Source: three-view drawing plus pictorial views. Frame: mm from the lowest corner of the part. Coordinates: 2 decimals unless noted, no trailing zeros. Loops run counter-clockwise (first coordinate to the right, second up) from the corner with the lowest first, then second, coordinate; pieces in that order, holes last. Notation, with made-up numbers: M 43,-1.75 L 100,-1.75 A13 cw 100,16.25 Z; hole C -19,75.5 d8. An arc over 180 degrees is marked long. Write each question's results on one line, items separated by ' | '. Start each with the question number.
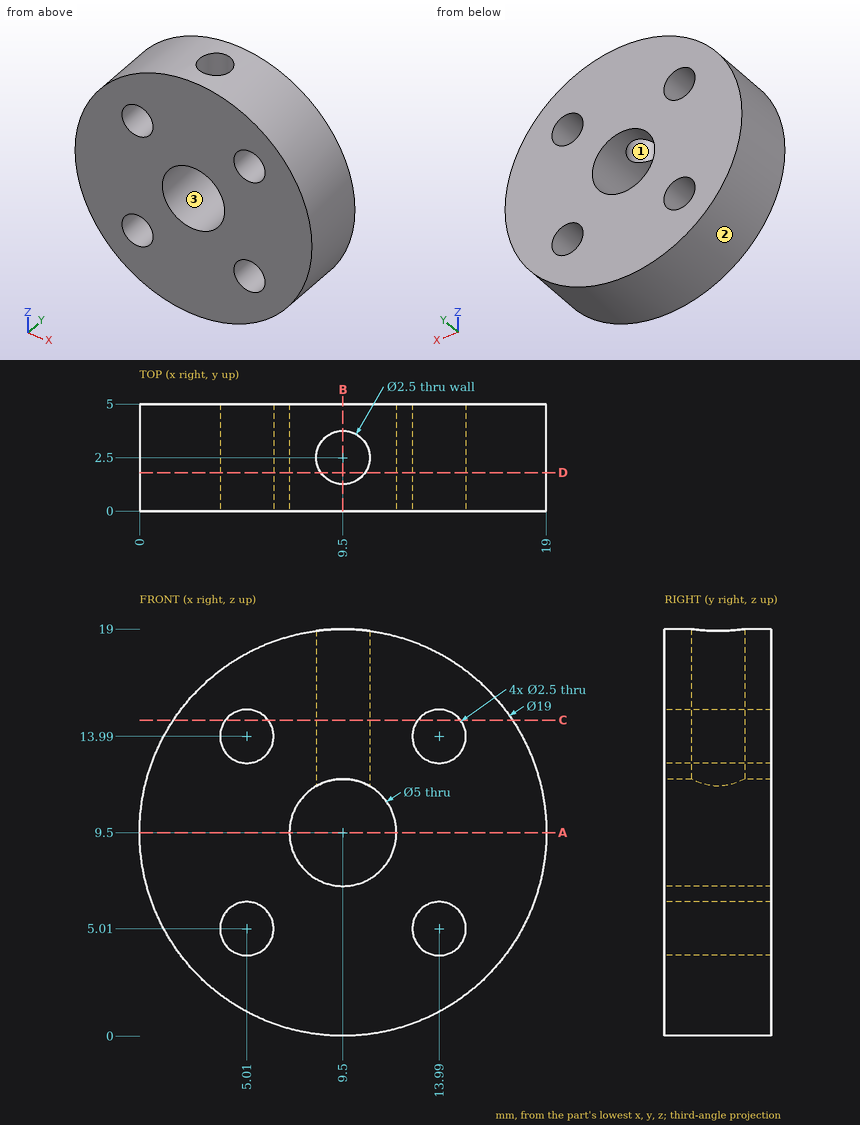
Item 1: Ray query, L1, parallel to Y at x = 9.5, z = 16.75; L2, parallel to X at y = 2.75, z = 5.75. Return the intervals inside material, ascending. Write a range as [from, to].
Item 2: Section D-D, the plane y = 1.8. Return loops of the section in (x, z), plus the area to 3 significant figures.
Item 3: Section B-B, the plane x = 9.5. Return loops of the section in (y, z), plus the area to 3 significant figures.
Item 4: Contact query for flat-ended pins moving along their axis: P1, Ø2, axis at x = 14.5, y = 4, coming from the +Z side; P2, Ø2, axis at x = 15.5, y = 1, coming from the +Z side. Output: stop coordinate, or through.
Item 5: Pull-direction query (Z, two-part tool) for the marked faces 1, 2 and 3; classes: released by +Z, released by -Z, zero draft, split by the parting line, or undercut.
Item 6: Section C-C, the plane z = 14.75. Return loops of the section in (x, y), plus the area to 3 significant figures.
Item 7: Section A-A, the plane z = 9.5. Return loops of the section in (x, y).
Solutions:
1) L1: y = [0, 1.25], [3.75, 5] | L2: x = [0.77, 4], [6.02, 12.98], [15, 18.23]
2) outline: M 8.46,11.78 L 8.46,18.94 A9.5 ccw long 10.54,18.94 L 10.54,11.78 A2.5 cw long Z; hole C 5.01,5.01 d2.5; hole C 5.01,13.99 d2.5; hole C 13.99,5.01 d2.5; hole C 13.99,13.99 d2.5 | area: 230 mm²
3) outline: M 0,0 L 5,0 L 5,7 L 0,7 Z; M 0,12 L 1.25,12 L 1.25,19 L 0,19 Z; M 3.75,12 L 5,12 L 5,19 L 3.75,19 Z | area: 52.5 mm²
4) P1: stops at z = 18.12 | P2: stops at z = 17.58
5) face 1: zero draft | face 2: split by the parting line | face 3: undercut
6) outline: M 1.58,0 L 4.02,0 L 4.02,5 L 1.58,5 Z; M 6,0 L 13,0 L 13,5 L 6,5 Z; M 14.98,0 L 17.42,0 L 17.42,5 L 14.98,5 Z; hole C 9.5,2.5 d2.5 | area: 54.4 mm²
7) outline: M 0,0 L 7,0 L 7,5 L 0,5 Z; M 12,0 L 19,0 L 19,5 L 12,5 Z
